from build123d import *

# Parameters (mm, degrees)
F1_W     = 32
F1_H     = 20
F2_DEPTH = 2
F3_W     = 22
F3_H     = 2
F3_W_2   = 2
F3_H_2   = 12
F4_DEPTH = 2
F5_W     = 2
F5_H     = 6
F6_DEPTH = 17


with BuildPart() as f2:
    # F1 (on Top) → F2 (new body)
    with BuildSketch(Plane.XY):
        Rectangle(F1_W, F1_H)
    extrude(amount=F2_DEPTH)

    # F3 (on face) → F4 (join)
    with BuildSketch(Plane.XY.offset(2)):
        with Locations((-1, 7)):
            Rectangle(F3_W, F3_H)
        with Locations((13, 2)):
            Rectangle(F3_W_2, F3_H_2)
        with Locations((1, -7)):
            Rectangle(F3_W, F3_H)
        with Locations((-13, -2)):
            Rectangle(F3_W_2, F3_H_2)
    extrude(amount=F4_DEPTH)

    # F5 (on face) → F6 (join)
    with BuildSketch(Plane.XY.offset(2)):
        with Locations((-9, 1)):
            Rectangle(F5_W, F5_H)
        Polygon((-10, -2), (-10, -4), (10, -4), (10, -2), (8, -2), (-8, -2), align=None)
        with Locations((9, 1)):
            Rectangle(F5_W, F5_H)
    extrude(amount=F6_DEPTH)


solid = f2.part
CAD build for the part. Positions are in the model's coordinates, mm. A direction names the side the tool comes from. Round coordinates to 2 decimals unless told otherwise and drop trailing zeros. Loops run counter-clockwise (first coordinate to the right, second up) from the corner with the lowest first, then second, coordinate; pieces in that order, holes last.
(1) Cut at B-B (x = 13.5). Give the cut face in (y, z), plus the area to 3 significant figures.
(2) Cut at C-C (y = 5). Give the cut face in (x, z).
(3) Two-plate mould, pull along X, no slides. Class faces 5 (the flat face through (13, 2, 4)), 6 (the flat face through (0, -2, 10)), 7 (the flat face through (-14, -2, 3)): +X half, -X half, draft (parallel to the pull), parting line (faces both ways), or undercut.
(4) Wall check: line 1 along Y through (x, z) = (1, 3.5); line 2 along Y through (x, z) = (9, 3.75); line 3 along X through (y, z) = (0.75, 2.5). Give the ranges that are in metal, low to high.
(5) Drop flat-ended pins along their axis: pin 1 (12 mm diameter, centred on x = -5.5, y = 0.5, fed in from -Z); pin 2 (1.8 mm diameter, centred on y = 2, z = 14, fed in from -X); pin 3 (1.6 mm diameter, centred on y = -1, z = 3, fed in from -X); pin 4 (1 mm diameter, centred on x = 5, z = 13.5, fed in from +Y). Give the stop position or say it passes through.
(6) Cut at D-D (y = -2.75). Give the cut face in (x, z), plus the area to 3 significant figures.
(7) Cut at A-A (z = 2.5). Give the cut face in (x, y).
(8) Which spindle directions (+Z, -Z, +X, -X, +Y, -Y) get a long thin tool onto all of the face, cutting with end or side? Do faces 1 (the flat face through (-12, 7, 3)), 2 (the flat face through (1, -8, 3)), 3 (the flat face through (-13, -2, 4)), 4 (the flat face through (14, 2, 3)). Say none if no direction does.
Findings below:
1. outline: (-10, 0) - (10, 0) - (10, 2) - (8, 2) - (8, 4) - (-4, 4) - (-4, 2) - (-10, 2) - close
1. area: 64.0 mm2
2. outline: (-16, 0) - (16, 0) - (16, 2) - (14, 2) - (14, 4) - (12, 4) - (12, 2) - (-16, 2) - close
3. face 5: draft
3. face 6: undercut
3. face 7: -X half
4. line 1: y = -8 to -6, -4 to -2, 6 to 8
4. line 2: y = -8 to -6, -4 to 4, 6 to 8
4. line 3: x = -14 to -12, -10 to -8, 8 to 10, 12 to 14
5. pin 1: stops at z = 0
5. pin 2: stops at x = -10
5. pin 3: stops at x = -14
5. pin 4: stops at y = -2
6. outline: (-16, 0) - (16, 0) - (16, 2) - (14, 2) - (14, 4) - (12, 4) - (12, 2) - (10, 2) - (10, 19) - (-10, 19) - (-10, 2) - (-12, 2) - (-12, 4) - (-14, 4) - (-14, 2) - (-16, 2) - close
6. area: 412 mm2
7. outline: (-14, -8) - (-12, -8) - (-12, 4) - (-14, 4) - close; (-12, 6) - (10, 6) - (10, 8) - (-12, 8) - close; (-10, -8) - (12, -8) - (12, -6) - (-10, -6) - close; (-10, -4) - (10, -4) - (10, 4) - (8, 4) - (8, -2) - (-8, -2) - (-8, 4) - (-10, 4) - close; (12, -4) - (14, -4) - (14, 8) - (12, 8) - close
8. face 1: +Z, -X, +Y
8. face 2: +Z, +X, -X, -Y
8. face 3: +Z, -X, +Y, -Y
8. face 4: +Z, +X, +Y, -Y
